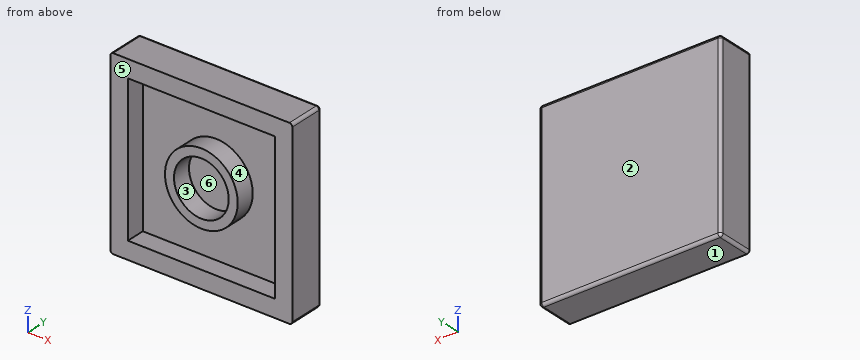
```python
from build123d import *

# Parameters (mm, degrees)
SKETCH2_W           = 15.875
SKETCH2_H           = 15.875
BOSS_EXTRUDE3_DEPTH = 3.175
SHELL1_T            = -1.524
SKETCH5_R           = 3.175
SKETCH5_R_2         = 2.3876
BOSS_EXTRUDE6_DEPTH = 1.651
FILLET1_R           = 0.254


with BuildPart() as part:
    # Sketch2 → Boss-Extrude3 (new body)
    with BuildSketch(Plane(origin=(0, 0, 0), x_dir=(1, 0, 0), z_dir=(0, 1, 0))):
        with Locations((-9.795613381, 0.785891089)):
            Rectangle(SKETCH2_W, SKETCH2_H)
    extrude(amount=BOSS_EXTRUDE3_DEPTH)

    # Shell1
    shell1_openings = [part.faces().sort_by_distance(p)[0] for p in [
        (-9.795613381, 0, -0.785891089),
    ]]
    offset(amount=SHELL1_T, openings=shell1_openings, kind=Kind.INTERSECTION)

    # Sketch5 → Boss-Extrude6 (add)
    with BuildSketch(Plane.XZ):
        with Locations((-9.795613381, -0.785891089)):
            Circle(SKETCH5_R)
        with Locations((-9.795613381, -0.785891089)):
            Circle(SKETCH5_R_2, mode=Mode.SUBTRACT)
    extrude(amount=-BOSS_EXTRUDE6_DEPTH)

    # Fillet1
    fillet1_edges = [part.edges().sort_by_distance(p)[0] for p in [
        (-1.858113381, 3.175, -0.785891089),
        (-9.795613381, 3.175, -8.723391089),
        (-17.733113381, 3.175, -0.785891089),
        (-17.733113381, 1.5875, -8.723391089),
        (-1.858113381, 1.5875, -8.723391089),
        (-1.858113381, 1.5875, 7.151608911),
        (-17.733113381, 1.5875, 7.151608911),
        (-9.795613381, 3.175, 7.151608911),
    ]]
    fillet(fillet1_edges, radius=FILLET1_R)


solid = part.part
```
The model under review builds one solid part; all positions refer to its coordinate system, in mm. Face numbers are marked on the shaded views. A direction names the side the tool comes from. Coordinates: 2 decimals unless noted, no trailing zeros. Write each loop counter-clockwise with the first axis right and the second up, starting at its lowest first coordinate (ties: lowest second). Pieces come first, ordered by that corner, then holes.
1) The part is to be moulded in two halves that separate along Z. For the marked faces 1, 2, 3 and 4, say which applies: pulls with the +Z half, pulls with the -Z half, needs draft (parallel to the pull), parting line crosses it, or undercut.
2) Machinability: for the marked faces 5 and 6, which of the approach directions +Z, -Z, +X, -X, +Y, -Y give a long, thin tool a straight path to every point of the face, cutting with its end or side? Answer none if there is none.
3) We need section B-B on z = -5.5. State the section outline as (x, y) points (3 decimals).
4) We need section D-D on z = -2.5. State the section outline as (x, y) points (3 decimals), then the cut area to 3 significant figures.
5) We need section A-A on y = 0.75. State the section outline as (x, z) points (3 decimals), then the cut area to 3 significant figures.
6) Clearance check with flat-ended pins moving along their axes: pin 1 Ø1.4 at (x, z) = (-11, -1.5) entering from -Y; pin 2 Ø2 at (x, z) = (-8.5, 5.5) entering from -Y. State where each tip first meets the part, or that it passes through.
7) We need section C-C on x = -4.5. State the section outline as (y, z) points (3 decimals).
8) To check wall thickness, follow probe 1 along Z at (x, y) = (-14.5, 1.1); probe 2 along X at (y, z) = (0.65, -5); probe 3 along X at (y, z) = (1.3, -3.5). State the ranges of each line that lie inside material, in increasing order.
Answer list:
1. face 1: pulls with the -Z half
1. face 2: needs draft
1. face 3: undercut
1. face 4: undercut
2. face 5: +Z, -Z, +X, -X, -Y
2. face 6: -Y
3. outline: (-17.733, 0) - (-16.209, 0) - (-16.209, 1.651) - (-3.382, 1.651) - (-3.382, 0) - (-1.858, 0) - (-1.858, 2.921) arc R0.254 ccw to (-2.112, 3.175) - (-17.479, 3.175) arc R0.254 ccw to (-17.733, 2.921) - close
4. outline: (-17.733, 0) - (-16.209, 0) - (-16.209, 1.651) - (-12.468, 1.651) - (-12.468, 0) - (-11.458, 0) - (-11.458, 1.651) - (-8.134, 1.651) - (-8.134, 0) - (-7.123, 0) - (-7.123, 1.651) - (-3.382, 1.651) - (-3.382, 0) - (-1.858, 0) - (-1.858, 2.921) arc R0.254 ccw to (-2.112, 3.175) - (-17.479, 3.175) arc R0.254 ccw to (-17.733, 2.921) - close
4. area: 32.5 mm2
5. outline: (-17.733, -8.469) arc R0.254 ccw to (-17.479, -8.723) - (-2.112, -8.723) arc R0.254 ccw to (-1.858, -8.469) - (-1.858, 6.898) arc R0.254 ccw to (-2.112, 7.152) - (-17.479, 7.152) arc R0.254 ccw to (-17.733, 6.898) - close; circle Ø6.35 at (-9.796, -0.786); hole (-16.209, -7.199) - (-3.382, -7.199) - (-3.382, 5.628) - (-16.209, 5.628) - close; hole circle Ø4.775 at (-9.796, -0.786)
5. area: 101 mm2
6. pin 1: stops at y = 1.65
6. pin 2: stops at y = 0
7. outline: (0, -8.723) - (2.921, -8.723) arc R0.254 ccw to (3.175, -8.469) - (3.175, 6.898) arc R0.254 ccw to (2.921, 7.152) - (0, 7.152) - (0, 5.628) - (1.651, 5.628) - (1.651, -7.199) - (0, -7.199) - close
8. probe 1: z = -8.72 to -7.2, 5.63 to 7.15
8. probe 2: x = -17.73 to -16.21, -3.38 to -1.86
8. probe 3: x = -17.73 to -16.21, -11.44 to -8.15, -3.38 to -1.86
